```python
from build123d import *

# Parameters (mm, degrees)
F1_DEPTH    = 7.5
F2_W        = 9.8101310167
F2_H        = 12.6
F3_DEPTH    = 2
F4_R        = 1.6
F5_T1_DEPTH = 20.0711055919


# Not quite as in the source:
# - a fillet or chamfer that OpenCascade refuses, or shapes differently, is made with other operations: its cross-section is extruded or revolved along the edge and cut away or added


with BuildPart() as f1:
    # F0 (on Top) → F1 (new body, symmetric)
    with BuildSketch(Plane.XY):
        with BuildLine():
            ThreePointArc((33.2014997867, 0.1693742672), (34.7428713669, 0.5269798189), (34.3852658153, 2.068351399))
            ThreePointArc((34.3852658153, 2.068351399), (0.2265050268, 11.9077038946), (-34, 2.3066544839))
            Line((-34, 2.3066544839), (-34, 0))
            Line((-34, 0), (-22.8898689833, 0))
            ThreePointArc((-22.8898689833, 0), (5.1340927179, 7.2785489292), (33.2014997867, 0.1693742672))
        make_face()
    extrude(amount=F1_DEPTH, both=True)

    # F2 (on Front) → F3 (cut)
    with BuildSketch(Plane.XZ):
        with Locations((-28.2949344917, 0)):
            Rectangle(F2_W, F2_H)
    extrude(amount=-F3_DEPTH, mode=Mode.SUBTRACT)

    # F4
    f4_edges = [f1.edges().sort_by_distance(p)[0] for p in [
        (-28.294934, 2, 6.3),
        (-33.2, 2, 0),
        (-28.294934, 2, -6.3),
        (-23.389869, 2, 0),
        (-34, 2.306654, 0),
        (-34, 1.153327, 7.5),
        (-34, 1.153327, -7.5),
    ]]
    fillet(f4_edges, radius=F4_R)

    # F5: fillet of radius 4 on 1 edges, made by hand

    # F5_s2 → F5_t1 (cut)
    with BuildSketch(Plane.XY.offset(-10.0355527959)):
        with BuildLine():
            ThreePointArc((-23.9040901017, 0), (-22.9370384998, 0.1186585825), (-22.0273613841, 0.4675944003))
            ThreePointArc((-22.0273613841, 0.4675944003), (-22.4595993901, 0.2356126314), (-22.8898689833, 0))
            Line((-22.8898689833, 0), (-23.9040901017, 0))
        make_face()
    extrude(amount=F5_T1_DEPTH, mode=Mode.SUBTRACT)


solid = f1.part
```
The listing builds one solid part. Answer for the finished solid, in the listing's coordinates (mm). A direction names the side the tool comes from. Coordinates: 2 decimals unless noted, no trailing zeros. Write each loop counter-clockwise with the first axis right and the second up, starting at its lowest first coordinate (ties: lowest second). Pieces come first, ordered by that corner, then holes. Notation, with made-up numbers: (32, 53.25) - (46, 53.25) arc R30 cw to (46, 92.25) - close; hole circle Ø11 at (-3.75, 14.5). An arc over 180 degrees is marked (long way). Return JSON: item names as keys, results as strings. Group by question number.
1. Determine the mould class of faces 4 (the flat face through (-7, 7, -7.5)), 5 (the cylindrical face through (1.181, 11.897, 0.105)), 6 (the cylindrical face through (-23.85, 1.52, 0.09)) for opening direction Z: released by +Z, released by -Z, zero draft, split by the parting line, or undercut.
2. Straight lines are drawn through the part: L1, parallel to Y at x = 21.5, z = -4; L2, parallel to X at y = 2.5, z = -6; L3, parallel to Y at x = -30.5, z = -5.75. For each, find the intervals that lie inside material, in ascending order.
3. A cutting plane is placed at A-A, the plane y = 6.5. Determine the outline of the cut face in (x, z).
4. Given pin 1 (4 mm diameter, centred on x = -15.5, z = -5, fed in from -Y); pin 2 (8 mm diameter, centred on x = 11.5, z = -4.5, fed in from -Y); pin 3 (6 mm diameter, centred on x = 10.5, y = 3, fed in from -Z); pin 4 (2 mm diameter, centred on y = 2.5, z = -5.5, fed in from +X), each flat-ended and moving along its own axis, determine where each tip first touches the part or whether it passes through.
5. Which of the six approach directions +Z, -Z, +X, -X, +Y, -Y give full straight-line access (tool end or side, diameter ignored) to faces 1 (the cylindrical face through (-28.23, 1.52, -5.84)), 2 (the cylindrical face through (-22.741, 0.173, -0.105)), 3 (the cylindrical face through (-33.303, 1.244, 7.221))?
6. A cutting plane is placed at D-D, the plane y = 9.75. Determine the outline of the cut face in (x, z), plus the area to 3 significant figures.
7. A cutting plane is placed at B-B, the plane z = -0.75. Determine the outline of the cut face in (x, y), plus the area to 3 significant figures.
8. A cutting plane is placed at C-C, the plane x = -28.5. Determine the outline of the cut face in (y, z).
Ans:
{
 "1": {"face 4": "released by -Z", "face 5": "zero draft", "face 6": "undercut"},
 "2": {"L1": "4.98 to 8.25", "L2": "-33.57 to -17.8, 28.42 to 33.68", "L3": "1.61 to 4.31"},
 "3": {"outline": "(-25.96, -7.5) - (-4.18, -7.5) - (-4.18, 7.5) - (-25.96, 7.5) - close; (14.8, -7.5) - (25.96, -7.5) - (25.96, 7.5) - (14.8, 7.5) - close"},
 "4": {"pin 1": "y = 2.63", "pin 2": "y = 6.38", "pin 3": "through", "pin 4": "x = 34.85"},
 "5": {"face 1": "-Y", "face 2": "+Z, -Z, -Y", "face 3": "+Z, -X, +Y, -Y"},
 "6": {"outline": "(-16.61, -7.5) - (16.61, -7.5) - (16.61, 7.5) - (-16.61, 7.5) - close", "area": "498 mm²"},
 "7": {"outline": "(-34, 0) - (-33.2, 0) - (-33.2, 0.4) arc R1.6 cw to (-31.6, 2) - (-24.99, 2) arc R1.6 cw to (-23.39, 0.4) - (-23.39, 0.03) arc R4 ccw to (-22.03, 0.47) arc R58.27 cw to (33.2, 0.17) arc R1.12 ccw to (34.39, 2.07) arc R65 ccw to (-33.22, 2.78) arc R1.6 ccw to (-34, 1.4) - close", "area": "304 mm²"},
 "8": {"outline": "(0, -7.5) - (5.33, -7.5) - (5.33, 7.5) - (0, 7.5) - (0, 6.3) - (0.4, 6.3) arc R1.6 cw to (2, 4.7) - (2, -4.7) arc R1.6 cw to (0.4, -6.3) - (0, -6.3) - close"}
}
